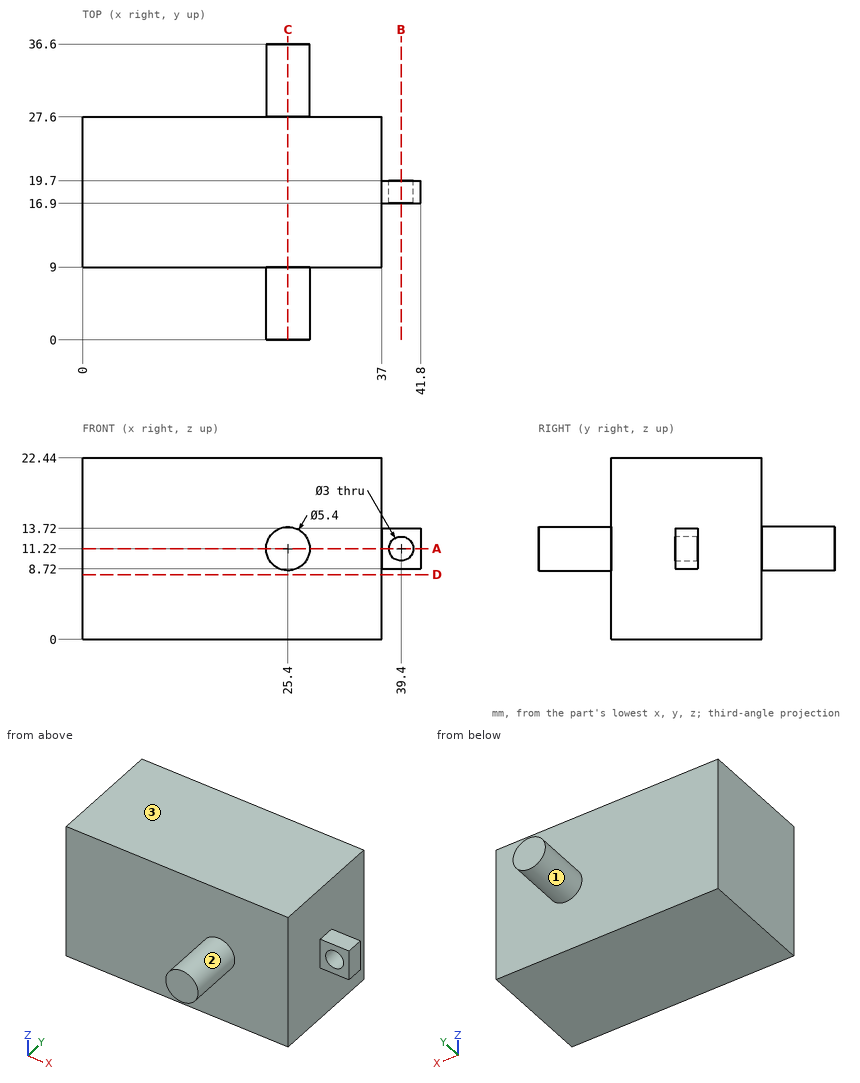
Geometry check sheet. Reference: drawing and pictorial views, mm from the part's lowest x, y, z. A direction names the side the tool comes from. Give positions to 0.01 mm unless a question says otherwise; leave off trailing zeros. Order: outer loops, then holes, each group sorted by start corner. A loop starts at its lowest first (then second) coordinate and runs counter-clockwise, first axis right, second up.
1. Section check D-D, the plane z = 8. Enter the section's corners in (x, y), and give its area (3 significant figures).
2. Section check A-A, the plane z = 11.22. Enter the section's corners in (x, y), and give its area (3 significant figures).
3. Section check C-C, the plane x = 25.4. Enter the section's corners in (y, z).
4. Thickness scan on L1, parallel to X at y = 18.35, z = 11.22; L2, parallel to Y at x = 12.5, z = 4; L3, parallel to Z at x = 39, y = 18. Record the ranges inside material, lowest first.
5. Access from +Z, -Z, +X, -X, +Y, -Y to the whole of each face (thin tool, end or side, straight path). Record for the marked faces 1, 2 and 3.
6. Section check B-B, the plane x = 39.4. Enter the section's corners in (y, z).
7. Gauge pin test, flat ends, axial feed: pin 1 Ø11 at (x, z) = (14, 13) entering from -Y; pin 2 Ø1.4 at (x, y) = (40, 19) entering from +Z; pin 3 Ø5 at (y, z) = (12, 9) entering from +X; pin 4 Ø1.5 at (x, y) = (10, 7.5) entering from -Z. Record the tip position at first contact, or that the pin passes through.
Values follow:
1. outline: (0, 9) - (37, 9) - (37, 27.6) - (0, 27.6) - close
1. area: 688 mm2
2. outline: (0, 9) - (22.7, 9) - (22.7, 0) - (28.1, 0) - (28.1, 9) - (37, 9) - (37, 16.9) - (37.9, 16.9) - (37.9, 19.7) - (37, 19.7) - (37, 27.6) - (28.1, 27.6) - (28.1, 36.6) - (22.7, 36.6) - (22.7, 27.6) - (0, 27.6) - close; (40.9, 16.9) - (41.8, 16.9) - (41.8, 19.7) - (40.9, 19.7) - close
2. area: 790 mm2
3. outline: (0, 8.52) - (9, 8.52) - (9, 0) - (27.6, 0) - (27.6, 8.52) - (36.6, 8.52) - (36.6, 13.92) - (27.6, 13.92) - (27.6, 22.44) - (9, 22.44) - (9, 13.92) - (0, 13.92) - close
4. L1: x = 0 to 37.9, 40.9 to 41.8
4. L2: y = 9 to 27.6
4. L3: z = 8.72 to 9.77, 12.67 to 13.72
5. face 1: +Y
5. face 2: -Y
5. face 3: +Z, +X, -X, +Y, -Y
6. outline: (16.9, 8.72) - (19.7, 8.72) - (19.7, 9.72) - (16.9, 9.72) - close; (16.9, 12.72) - (19.7, 12.72) - (19.7, 13.72) - (16.9, 13.72) - close
7. pin 1: stops at y = 9
7. pin 2: stops at z = 13.72
7. pin 3: stops at x = 37
7. pin 4: passes through
